Model file for the job. Use its own axes, mm. A direction names the side the tool comes from. Round coordinates to 2 decimals unless told otherwise and drop trailing zeros. Order: outer loops, then holes, each group sorted by start corner. A loop starts at its lowest first (then second) coordinate and runs counter-clockwise, first axis right, second up. Notation, with made-up numbers: (82.25, 4.5) -> (101.25, 4.5) arc R10 ccw to (101.25, 18.5) -> close; hole circle Ø3 at (-40, -37). An arc over 180 degrees is marked (long way). Use CSV: the item, a comma, the result in double quotes.
```python
from build123d import *

# Parameters (mm, degrees)
SKETCH1_R           = 31.75
SKETCH1_R_2         = 12.827
BOSS_EXTRUDE1_DEPTH = 5.1054
SKETCH2_R           = 31.75
SKETCH2_R_2         = 5.715
BOSS_EXTRUDE2_DEPTH = 14.224
CHAMFER1_SIZE       = 5.08
CHAMFER2_SIZE       = 12.7


with BuildPart() as part:
    # Sketch1 → Boss-Extrude1 (new body)
    with BuildSketch(Plane(origin=(0, 0, 0), x_dir=(1, 0, 0), z_dir=(0, 1, 0))):
        Circle(SKETCH1_R)
        Circle(SKETCH1_R_2, mode=Mode.SUBTRACT)
    extrude(amount=BOSS_EXTRUDE1_DEPTH)

    # Sketch2 → Boss-Extrude2 (add)
    with BuildSketch(Plane(origin=(0, 5.1054, 0), x_dir=(1, 0, 0), z_dir=(0, 1, 0))):
        Circle(SKETCH2_R)
        Circle(SKETCH2_R_2, mode=Mode.SUBTRACT)
    extrude(amount=BOSS_EXTRUDE2_DEPTH)

    # Chamfer1
    chamfer1_edges = [part.edges().sort_by_distance(p)[0] for p in [
        (-12.827, 0, 0),
    ]]
    chamfer(chamfer1_edges, length=CHAMFER1_SIZE)

    # Chamfer2
    chamfer2_edges = [part.edges().sort_by_distance(p)[0] for p in [
        (-31.75, 19.3294, 0),
    ]]
    chamfer(chamfer2_edges, length=CHAMFER2_SIZE)


solid = part.part
```
Q1. Cut at B-B (x = 0). Give the cut face in (y, z) (3 decimals), plus the area to 3 significant figures.
From the geometry:
outline,"(0, -31.75) -> (6.629, -31.75) -> (19.329, -19.05) -> (19.329, -5.715) -> (5.105, -5.715) -> (5.105, -12.827) -> (5.08, -12.827) -> (0, -17.907) -> close; (0, 17.907) -> (5.08, 12.827) -> (5.105, 12.827) -> (5.105, 5.715) -> (19.329, 5.715) -> (19.329, 19.05) -> (6.629, 31.75) -> (0, 31.75) -> close"
area,"747 mm²"
Q2. Mould opens along X. For faces 3 (the conical face through (-4.26, 18.71, 19.2)), 4 (the flat face through (4, 19.329, -5)), 5 (the conical face through (-1.702, 4.833, -12.962)) say: +X half, -X half, draft (parallel to the pull), parting line (faces both ways), or undercut.
From the geometry:
face 3,"parting line"
face 4,"draft"
face 5,"undercut"
Q3. Probe line 1 along X through (y, z) = (5.15, 0) (3 decimals); line 2 along X through (y, z) = (13, -1.5); line 3 along Z through (x, y) = (0, 11.75) (3 decimals). List the from-to ranges inside material, lowest first.
From the geometry:
line 1,"x = -31.75 to -5.715, 5.715 to 31.75"
line 2,"x = -25.34 to -5.51, 5.51 to 25.34"
line 3,"z = -26.629 to -5.715, 5.715 to 26.629"
Q4. Cut at D-D (y = 9.5). Give the cut face in (x, z) (3 decimals), plus the area to 3 significant figures.
From the geometry:
outline,"circle Ø57.759 at (0, 0); hole circle Ø11.43 at (0, 0)"
area,"2,520 mm²"
Q5. Cut at C-C (y = 13.75). Give the cut face in (x, z) (3 decimals), plus the area to 3 significant figures.
From the geometry:
outline,"circle Ø49.259 at (0, 0); hole circle Ø11.43 at (0, 0)"
area,"1,800 mm²"
Q6. Cut at A-A (z = 0). Give the cut face in (x, y) (3 decimals), plus the area to 3 significant figures.
From the geometry:
outline,"(-31.75, 0) -> (-17.907, 0) -> (-12.827, 5.08) -> (-12.827, 5.105) -> (-5.715, 5.105) -> (-5.715, 19.329) -> (-19.05, 19.329) -> (-31.75, 6.629) -> close; (5.715, 5.105) -> (12.827, 5.105) -> (12.827, 5.08) -> (17.907, 0) -> (31.75, 0) -> (31.75, 6.629) -> (19.05, 19.329) -> (5.715, 19.329) -> close"
area,"747 mm²"
Q7. Pin check, flat tips, straight feed: pin 1 (4 mm diameter, centred on x = 5.5, y = 6, fed in from +Z); pin 2 (1.5 mm diameter, centred on x = -3, y = 10.5, fed in from -Z); pin 3 (6 mm diameter, centred on x = -25, y = 3.5, fed in from +Z). Stop position of each tip, or through.
From the geometry:
pin 1,"stops at z = 31.56"
pin 2,"stops at z = -28.48"
pin 3,"stops at z = 22.89"
Q8. Which spindle directions (+Z, -Z, +X, -X, +Y, -Y) get a long thin tool onto all of the face, cutting with end or side? Do faces 1 (the flat face through (3, 5.105, 6)), 2 (the cylindrical face through (-6.883, 3.268, 30.995)). Say none if no direction does.
From the geometry:
face 1,"-Y"
face 2,"+Y, -Y"
